```python
from build123d import *

# Parameters (mm, degrees)
SKETCH1_W                      = 100
SKETCH1_H                      = 100
SKETCH1_W_2                    = 94
SKETCH1_H_2                    = 94
EXTRUDE_THIN1_DEPTH            = 130
FILLET1_R                      = 0.5
FILLET2_R                      = 3
F_8_0_8_DIAMETER_HOLE2_D       = 8
F_8_0_8_DIAMETER_HOLE3_D       = 8
F_10_0_10_DIAMETER_HOLE1_D     = 10
F_10_0_10_DIAMETER_HOLE2_D     = 10
F_21_0_21_DIAMETER_HOLE1_D     = 42
F_21_0_21_DIAMETER_HOLE1_DEPTH = 3
F_5_0_5_DIAMETER_HOLE1_D       = 5
F_5_0_5_DIAMETER_HOLE1_DEPTH   = 3
F_8_0_8_DIAMETER_HOLE5_D       = 8
F_8_0_8_DIAMETER_HOLE5_DEPTH   = 3
CUT_EXTRUDE1_REACH             = 173.464
SKETCH34_R                     = 2
SKETCH35_R                     = 2
CUT_EXTRUDE2_DEPTH             = 10
SKETCH36_R                     = 2
CUT_EXTRUDE3_DEPTH             = 10
SKETCH37_R                     = 2
CUT_EXTRUDE4_DEPTH             = 10
SKETCH38_R                     = 3.1
CUT_EXTRUDE5_DEPTH             = 10
SKETCH39_R                     = 3.1
CUT_EXTRUDE6_DEPTH             = 10


with BuildPart() as part:
    # Sketch1 → Extrude-Thin1 (new body)
    with BuildSketch(Plane.XY):
        Rectangle(SKETCH1_W, SKETCH1_H)
        Rectangle(SKETCH1_W_2, SKETCH1_H_2, mode=Mode.SUBTRACT)
    extrude(amount=EXTRUDE_THIN1_DEPTH)

    # Fillet1
    fillet1_edges = [part.edges().sort_by_distance(p)[0] for p in [
        (47, -47, 65),
        (47, 47, 65),
        (-47, 47, 65),
        (-47, -47, 65),
    ]]
    fillet(fillet1_edges, radius=FILLET1_R)

    # Fillet2
    fillet2_edges = [part.edges().sort_by_distance(p)[0] for p in [
        (50, -50, 65),
        (-50, -50, 65),
        (-50, 50, 65),
        (50, 50, 65),
    ]]
    fillet(fillet2_edges, radius=FILLET2_R)

    # Ø8.0 (8) Diameter Hole2 (through all)
    with Locations(Plane(origin=(0, 50, 0), x_dir=(1, 0, 0), z_dir=(0, 1, 0))):
        with Locations((28, -32), (28, -90)):
            Hole(F_8_0_8_DIAMETER_HOLE2_D / 2)

    # Ø8.0 (8) Diameter Hole3 (through all)
    with Locations(Plane(origin=(50, 0, 0), x_dir=(0, 0, -1), z_dir=(1, 0, 0))):
        with Locations((-14, 31), (-116, 31)):
            Hole(F_8_0_8_DIAMETER_HOLE3_D / 2)

    # Ø10.0 (10) Diameter Hole1 (through all)
    with Locations(Plane(origin=(0, 50, 0), x_dir=(1, 0, 0), z_dir=(0, 1, 0))):
        with Locations((-34, -56)):
            Hole(F_10_0_10_DIAMETER_HOLE1_D / 2)

    # Ø10.0 (10) Diameter Hole2 (through all)
    with Locations(Plane(origin=(50, 0, 0), x_dir=(0, 0, -1), z_dir=(1, 0, 0))):
        with Locations((-44, -31)):
            Hole(F_10_0_10_DIAMETER_HOLE2_D / 2)

    # Ø21.0 (21) Diameter Hole1
    with Locations(Plane(origin=(50, 0, 0), x_dir=(0, 0, -1), z_dir=(1, 0, 0))):
        with Locations((-70, 0)):
            Hole(F_21_0_21_DIAMETER_HOLE1_D / 2, depth=F_21_0_21_DIAMETER_HOLE1_DEPTH)

    # Ø5.0 (5) Diameter Hole1
    with Locations(Plane(origin=(50, 0, 0), x_dir=(0, 0, -1), z_dir=(1, 0, 0))):
        with Locations((-41.157258279, -16.652364697), (-53.347635303, 28.842741721), (-98.842741721, 16.652364697), (-86.652364697, -28.842741721)):
            Hole(F_5_0_5_DIAMETER_HOLE1_D / 2, depth=F_5_0_5_DIAMETER_HOLE1_DEPTH)

    # Ø8.0 (8) Diameter Hole5
    with Locations(Plane(origin=(0, 50, 0), x_dir=(1, 0, 0), z_dir=(0, 1, 0))):
        with Locations((-3, -25)):
            Hole(F_8_0_8_DIAMETER_HOLE5_D / 2, depth=F_8_0_8_DIAMETER_HOLE5_DEPTH)

    # Sketch34 → Cut-Extrude1 (cut, up to next)
    with BuildSketch(Plane(origin=(0, 50, 0), x_dir=(1, 0, 0), z_dir=(0, 1, 0)), mode=Mode.PRIVATE) as cut_extrude1_sk1:
        with Locations(Location((-22, -14, 0), (0, 0, 270))):
            Circle(SKETCH34_R)
    cut_extrude1_tool1 = extrude(cut_extrude1_sk1.sketch, amount=-CUT_EXTRUDE1_REACH, mode=Mode.PRIVATE) & part.part
    # Sketch34 → Cut-Extrude1 (cut, up to next)
    with BuildSketch(Plane(origin=(0, 50, 0), x_dir=(1, 0, 0), z_dir=(0, 1, 0)), mode=Mode.PRIVATE) as cut_extrude1_sk2:
        with Locations(Location((-11, -14, 0), (0, 0, 270))):
            Circle(SKETCH34_R)
    cut_extrude1_tool2 = extrude(cut_extrude1_sk2.sketch, amount=-CUT_EXTRUDE1_REACH, mode=Mode.PRIVATE) & part.part
    # Sketch34 → Cut-Extrude1 (cut, up to next)
    with BuildSketch(Plane(origin=(0, 50, 0), x_dir=(1, 0, 0), z_dir=(0, 1, 0)), mode=Mode.PRIVATE) as cut_extrude1_sk3:
        with Locations(Location((-11, -116, 0), (0, 0, 90))):
            Circle(SKETCH34_R)
    cut_extrude1_tool3 = extrude(cut_extrude1_sk3.sketch, amount=-CUT_EXTRUDE1_REACH, mode=Mode.PRIVATE) & part.part
    # Sketch34 → Cut-Extrude1 (cut, up to next)
    with BuildSketch(Plane(origin=(0, 50, 0), x_dir=(1, 0, 0), z_dir=(0, 1, 0)), mode=Mode.PRIVATE) as cut_extrude1_sk4:
        with Locations(Location((-22, -116, 0), (0, 0, 90))):
            Circle(SKETCH34_R)
    cut_extrude1_tool4 = extrude(cut_extrude1_sk4.sketch, amount=-CUT_EXTRUDE1_REACH, mode=Mode.PRIVATE) & part.part
    add(cut_extrude1_tool1.solids().sort_by_distance((-22, 50, 14))[0], mode=Mode.SUBTRACT)
    add(cut_extrude1_tool2.solids().sort_by_distance((-11, 50, 14))[0], mode=Mode.SUBTRACT)
    add(cut_extrude1_tool3.solids().sort_by_distance((-11, 50, 116))[0], mode=Mode.SUBTRACT)
    add(cut_extrude1_tool4.solids().sort_by_distance((-22, 50, 116))[0], mode=Mode.SUBTRACT)

    # Sketch35 → Cut-Extrude2 (cut)
    with BuildSketch(Plane.XZ.offset(50)):
        with Locations(Location((16, 44, 0), (0, 0, 270))):
            Circle(SKETCH35_R)
        with Locations(Location((5, 44, 0), (0, 0, 270))):
            Circle(SKETCH35_R)
    extrude(amount=-CUT_EXTRUDE2_DEPTH, mode=Mode.SUBTRACT)

    # Sketch36 → Cut-Extrude3 (cut)
    with BuildSketch(Plane.ZY.offset(50)):
        with Locations(Location((56, 19, 0), (0, 0, 270))):
            Circle(SKETCH36_R)
        with Locations(Location((56, 8, 0), (0, 0, 270))):
            Circle(SKETCH36_R)
    extrude(amount=-CUT_EXTRUDE3_DEPTH, mode=Mode.SUBTRACT)

    # Sketch37 → Cut-Extrude4 (cut)
    with BuildSketch(Plane(origin=(50, 0, 0), x_dir=(0, 0, -1), z_dir=(1, 0, 0))):
        with Locations(Location((-94, -19, 0), (0, 0, 90))):
            Circle(SKETCH37_R)
        with Locations(Location((-32, -19, 0), (0, 0, 90))):
            Circle(SKETCH37_R)
        with Locations(Location((-94, -8, 0), (0, 0, 90))):
            Circle(SKETCH37_R)
        with Locations(Location((-32, -9.079681112, 0), (0, 0, 90))):
            Circle(SKETCH37_R)
    extrude(amount=-CUT_EXTRUDE4_DEPTH, mode=Mode.SUBTRACT)

    # Sketch38 → Cut-Extrude5 (cut)
    with BuildSketch(Plane.ZY.offset(50)):
        with Locations(Location((56, 35, 0), (0, 0, 270))):
            Circle(SKETCH38_R)
        with Locations(Location((56, -15, 0), (0, 0, 270))):
            Circle(SKETCH38_R)
    extrude(amount=-CUT_EXTRUDE5_DEPTH, mode=Mode.SUBTRACT)

    # Sketch39 → Cut-Extrude6 (cut)
    with BuildSketch(Plane.XZ.offset(50)):
        with Locations(Location((-20, 44, 0), (0, 0, 270))):
            Circle(SKETCH39_R)
        with Locations(Location((35, 44, 0), (0, 0, 270))):
            Circle(SKETCH39_R)
    extrude(amount=-CUT_EXTRUDE6_DEPTH, mode=Mode.SUBTRACT)


solid = part.part
```
Geometry check sheet. Reference: the model listing, model coordinates, mm. A direction names the side the tool comes from. Round coordinates to 2 decimals unless told otherwise and drop trailing zeros. Order: outer loops, then holes, each group sorted by start corner. A loop starts at its lowest first (then second) coordinate and runs counter-clockwise, first axis right, second up. Notation, with made-up numbers: (46, 38) - (51, 38) arc R5 ccw to (51, 44) - close; hole circle Ø8 at (-22.75, -2). An arc over 180 degrees is marked (long way). Use a Markdown table: item, result. Add a question column.
1) Section check C-C (y = -34). Record the cut outline in (x, z).
2) Mould release check, pull along X, two halves, no side actions. Record for faces 6 (the cylindrical face through (49, -19, 96)), 7 (the cylindrical face through (28.867, -48.521, 93.905)), 8 (the cylindrical face through (28.521, -48.521, 28.034)), 9 (the flat face through (50, -11, 50)): released by +X, released by -X, zero draft, split by the parting line, or undercut.
3) Gauge pin test, flat ends, axial feed: P1, Ø9, axis at x = 28, z = 32, coming from the -Y side; P2, Ø3, axis at y = -9.08, z = 32, coming from the +X side. Record the tip position at first contact, or that the pin passes through.
4) Section check A-A (x = -27). Record the cut outline in (y, z).
5) Set-up check for faces 1 (the cylindrical face through (37.61, -48.52, 42.33)), 2 (the cylindrical face through (-2.479, 48.479, 21.034)), 3 (the cylindrical face through (48.479, -19.093, 40.615)), 4 (the cylindrical face through (-49, 19, 58)), 5 (the flat face through (-1, 50, 64)): record each of +Z, -Z, +X, -X, +Y, -Y from which the full face is reachable in a straight line by a thin tool's end or side.
6) Section check D-D (x = 35). Record the cut outline in (y, z).
7) Section check B-B (z = 116). Count the separate pieces of the cut face and the enclosed holes in it, then the cut area to 3 significant figures.
8) Thickness scan on line 1 along X through (y, z) = (-16.5, 28); line 2 along X through (y, z) = (-48.2, 44). Record the ranges inside material, lowest first.
Established:
| question | item | result |
|---|---|---|
| 1 | outline | (-50, 0) - (-47, 0) - (-47, 40) - (-50, 40) - close; (-50, 48) - (-47, 48) - (-47, 130) - (-50, 130) - close; (47, 0) - (50, 0) - (50, 40) - (47, 40) - close; (47, 48) - (50, 48) - (50, 130) - (47, 130) - close |
| 2 | face 6 | zero draft |
| 2 | face 7 | undercut |
| 2 | face 8 | undercut |
| 2 | face 9 | released by +X |
| 3 | P1 | y = -50 |
| 3 | P2 | x = -47 |
| 4 | outline | (-50, 0) - (-47, 0) - (-47, 130) - (-50, 130) - close; (47, 0) - (50, 0) - (50, 130) - (47, 130) - close |
| 5 | face 1 | -Y |
| 5 | face 2 | +Y |
| 5 | face 3 | +X |
| 5 | face 4 | -X |
| 5 | face 5 | +Z, -Z, +X, -X, +Y |
| 6 | outline | (-50, 0) - (-47, 0) - (-47, 40.9) - (-50, 40.9) - close; (-50, 47.1) - (-47, 47.1) - (-47, 130) - (-50, 130) - close; (47, 0) - (50, 0) - (50, 130) - (47, 130) - close |
| 7 | separate pieces | 4 |
| 7 | enclosed holes | 0 |
| 7 | area | 1,080 mm2 |
| 8 | line 1 | -50 to -47, 47 to 50 |
| 8 | line 2 | -49.75 to -23.1, -16.9 to 3, 7 to 14, 18 to 31.9, 38.1 to 49.75 |
